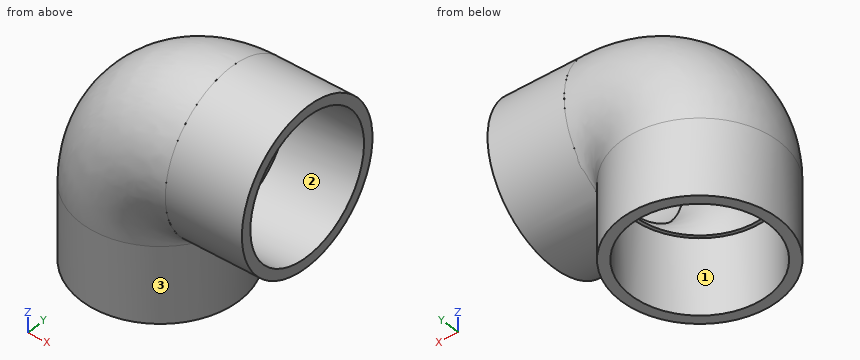
Autodesk Inventor part; units mm, degrees
ref_plane "YZ Plane" through (0, 0, 0) normal (1, 0, 0) x (0, 1, 0)
ref_plane "XZ Plane" through (0, 0, 0) normal (0, 1, 0) x (-1, 0, 0)
ref_plane "XY Plane" through (0, 0, 0) normal (0, 0, 1) x (1, 0, 0)
sketch "Sketch1" plane through (0, 0, 0) normal (0, 1, 0) x (-1, 0, 0)
  line L0 (0, 0) -> (0, 117) construction
  line L1 (0, 117) -> (-117, 117) construction
  line L2 (63.2, 0) -> (55, 0)
  line L3 (55, 0) -> (55, 61)
  line L4 (55, 61) -> (63.2, 61)
  line L5 (63.2, 61) -> (63.2, 0)
  line L6 (0, 0) -> (55, 0) construction
  line L7 (55, 61) -> (0, 61) construction
  line L8 (-117, 117) -> (-117, 172) construction
  line L9 (-117, 172) -> (-56, 172)
  line L10 (-56, 172) -> (-56, 180.2)
  line L11 (-56, 180.2) -> (-117, 180.2)
  line L12 (-117, 180.2) -> (-117, 172)
  line L13 (-56, 172) -> (-56, 117) construction
  dimension "d0" = 61
  dimension "d1" = 56
  dimension "d2" = 110
  dimension "d3" = 8.2
  dimension "d4" = 61
  dimension "d5" = 8.2
  dimension "d6" = 110
  dimension "d7" = 56
revolve "Revolution1" add sketch "Sketch1" angle 360 about axis through (0, 0, 117) along (1, 0, 0) contours L12 L11 L10 L9
revolve "Revolution2" add sketch "Sketch1" angle 360 about axis through (0, 0, 0) along (0, 0, 1) contours L2 L3 L4 L5
sketch "Sketch2" plane through (0, 0, 61) normal (0, 0, 1) x (1, 0, 0)
  line L0 (56, 29.295733) -> (56, -29.295733)
  line L1 (56, -29.295733) -> (56, 29.295733)
  line L2 (56, 55) -> (56, -55)
  line L3 (55.99, -29.314841) -> (55.99, 29.314841)
  arc A0 (56, 29.295733) -> (56, -29.295733) centre (0, 0) ccw
  circle A1 centre (0, 0) radius 63.2
  circle A2 centre (0, 0) radius 52.25
  dimension "d8" = 0.01
  dimension "d9" = 126.4
  dimension "d10" = 104.5
revolve "Revolution3" add sketch "Sketch2" angle 90 about axis through (55.99, -29.314841, 61) along (0, 1, 0) contours L3 A0
equation "\"d0\" = t1"
equation "\"d1\" = z1"
equation "\"d2\" = dd1"
equation "\"d3\" = s1"
equation "\"d4\" = t1"
equation "\"d5\" = s1"
equation "\"d6\" = dd1"
equation "\"d7\" = z1"
equation "\"d9\" = dd1 + 2 * s1"
equation "\"d10\" = 0.95 * dd1"
equation "\"z1\" = 56"
equation "\"t1\" = 61"
equation "\"s1\" = 8.2"
equation "\"dd1\" = 110"
properties part number "DIN 8063 Колено 90 градусов, тип W1 110" material "ПВХ, непластифицированный"
Work out the finished part from the listing and answer in its coordinate system (mm). Face numbers are marked on the shaded views. Coordinates: 2 decimals unless noted, no trailing zeros. Loops run counter-clockwise (first coordinate to the right, second up) from the corner with the lowest first, then second, coordinate; pieces in that order, holes last. Notation, with made-up numbers: (-24.75, 78.25) -> (13.25, 78.25) arc R19 ccw to (13.25, 109.25) -> close; hole circle Ø11 at (65.25, -18.5). An arc over 180 degrees is marked (long way). Write each question's results on one line, items separated by ' | '. Start each with the question number.
1) Flat-ended cylindrical pins translate along their axes: P1, Ø3, axis at x = 79, z = 51.5, coming from the -Y side; P2, Ø3, axis at x = 54, y = -17, coming from the +Z side; P3, Ø8, axis at y = 20.5, z = 143.5, coming from the +X side (3 decimals); P4, Ø12, axis at x = 38, y = -6, coming from the -Z side. Find the tip coordinate at first contact, or state that the pin passes through.
2) Find section C-C on z = 28. Determine the outline of the cut face in (x, y), then the cut area to 3 significant figures.
3) Consider line 1 along Y through (x, z) = (0, 18); line 2 along Z through (x, y) = (81, 0). Determine where each line is inside the solid, lowest interval first.
4) The mould has two halves that part along X. Classify the marked faces 1, 2 and 3: pulls with the +X half, pulls with the -X half, needs draft (parallel to the pull), parting line crosses it, or undercut.
5) Find section A-A on y = 0. Count the separate pieces of the cut face and the enclosed holes in it, then the cut area to 3 significant figures.
Response values:
1) P1: passes through | P2: stops at z = 178.24 | P3: stops at x = -1.015 | P4: stops at z = 165.9
2) outline: circle Ø126.4 at (0, 0); hole circle Ø110 at (0, 0) | area: 3,040 mm^2
3) line 1: y = -63.2 to -55, 55 to 63.2 | line 2: z = 53.8 to 62, 172 to 180.2
4) face 1: undercut | face 2: needs draft | face 3: parting line crosses it
5) separate pieces: 3 | enclosed holes: 0 | area: 3,920 mm^2
